from build123d import *

# Parameters (mm, degrees)
SKETCH1_W            = 94
SKETCH1_H            = 190
PLATE_DEPTH          = 12
SKETCH2_R            = 17.5
BOSS_DEPTH           = 10
SKETCH3_R            = 11
CENTER_HOLE_DEPTH    = 23
FILLET_R5_R          = 5
FILLET_R2_R          = 2
LPATTERN1_COUNT      = 5
LPATTERN1_PITCH      = 40
LPATTERN1_COUNT_DIR2 = 2
LPATTERN1_PITCH_DIR2 = 70
LPATTERN2_COUNT      = 2
LPATTERN2_PITCH      = 35


with BuildPart() as part:
    # Sketch1 → plate (new body)
    with BuildSketch(Plane(origin=(0, 0, 0), x_dir=(1, 0, 0), z_dir=(0, 1, 0))):
        Rectangle(SKETCH1_W, SKETCH1_H)
    extrude(amount=PLATE_DEPTH)

    # Sketch2 → boss (add)
    with BuildSketch(Plane(origin=(0, 12, 0), x_dir=(-1, 0, 0), z_dir=(0, 1, 0))):
        Circle(SKETCH2_R)
    extrude(amount=BOSS_DEPTH)

    # Sketch3 → center hole (cut, through all)
    with BuildSketch(Plane(origin=(0, 22, 0), x_dir=(-1, 0, 0), z_dir=(0, 1, 0))):
        Circle(SKETCH3_R)
    extrude(amount=-CENTER_HOLE_DEPTH, mode=Mode.SUBTRACT)

    # Sketch4 → pattern hole (revolve, cut)
    with BuildSketch(Plane(origin=(-35, 12, 80), x_dir=(0, 0, 1), z_dir=(1, 0, 0))):
        Polygon((0, 0), (0, 12), (4, 12), (4, 6.201721238), (6, 5), (6, 0), align=None)
    pattern_hole = revolve(axis=Axis((-35, 18.130023899, 80), (0, -1, 0)), mode=Mode.SUBTRACT)

    # Fillet R5
    fillet_r5_edges = [part.edges().sort_by_distance(p)[0] for p in [
        (-47, 6, -95),
        (47, 6, -95),
        (47, 6, 95),
        (-47, 6, 95),
    ]]
    fillet(fillet_r5_edges, radius=FILLET_R5_R)

    # Fillet R2
    fillet_r2_edges = [part.edges().sort_by_distance(p)[0] for p in [
        (17.5, 12, 0),
        (17.5, 22, 0),
        (47, 12, 0),
        (0, 12, 95),
        (-47, 12, 0),
        (0, 12, -95),
        (45.535533906, 12, -93.535533906),
        (-45.535533906, 12, -93.535533906),
        (-45.535533906, 12, 93.535533906),
        (45.535533906, 12, 93.535533906),
    ]]
    fillet(fillet_r2_edges, radius=FILLET_R2_R)

    # LPattern1: pattern hole 5 × 2
    with Locations(*[(j * LPATTERN1_PITCH_DIR2, 0, -i * LPATTERN1_PITCH) for i in range(LPATTERN1_COUNT) for j in range(LPATTERN1_COUNT_DIR2) if (i, j) != (0, 0)]):
        add(pattern_hole, mode=Mode.SUBTRACT)

    # LPattern2: pattern hole ×2
    with Locations(*[(i * LPATTERN2_PITCH, 0, 0) for i in range(1, LPATTERN2_COUNT)]):
        add(pattern_hole, mode=Mode.SUBTRACT)

    # LPattern3 copy 1 sketch → LPattern3 copy 1 (revolve, cut)
    with BuildSketch(Plane(origin=(0, 12, -80), x_dir=(0, 0, 1), z_dir=(1, 0, 0))):
        Polygon((0, 0), (0, 12), (4, 12), (4, 6.201721238), (6, 5), (6, 0), align=None)
    revolve(axis=Axis((0, 18.130023899, -80), (0, -1, 0)), mode=Mode.SUBTRACT)

    # LPattern3 copy 2 sketch → LPattern3 copy 2 (revolve, cut)
    with BuildSketch(Plane(origin=(-35, 12, -80), x_dir=(0, 0, 1), z_dir=(1, 0, 0))):
        Polygon((0, 0), (0, 12), (4, 12), (4, 6.201721238), (6, 5), (6, 0), align=None)
    revolve(axis=Axis((-35, 18.130023899, -80), (0, -1, 0)), mode=Mode.SUBTRACT)


solid = part.part
Read the model definition and answer for the solid it produces. Units are mm, in the model's axes. A direction names the side the tool comes from. Give positions to 0.01 mm unless a question says otherwise; leave off trailing zeros. Loops run counter-clockwise (first coordinate to the right, second up) from the corner with the lowest first, then second, coordinate; pieces in that order, holes last. Notation, with made-up numbers: (3.5, 75) - (18.5, 75) arc R18 cw to (18.5, 100) - close; hole circle Ø3 at (47.5, 54.5). An arc over 180 degrees is marked (long way). Answer as CSV lines item,"result". Start each with the question number.
1) Find section C-C (z = -40). Write down the section's boundary in (x, y).
2) Which of the six approach directions +Z, -Z, +X, -X, +Y, -Y give full straight-line access (tool end or side, diameter ignored) to faces 4 (the face through (40.857, 9.535, -41.301)), 5 (the face through (31.034, 2.94, 39.479))?
3) Determine the mould class of faces 1 (the face through (-1, 12, -22)), 2 (the face through (31.034, 2.94, -40.521)), 3 (the face through (45, 5, 94)) for opening direction Z: released by +Z, released by -Z, zero draft, split by the parting line, or undercut.
4) Find section A-A (z = 0). State how many separate pieces and enclosed holes the cut face has, then the cut area to 3 significant figures.
5) Each of these flat-tipped pins is pushed along its axis until it touches: pin 1 Ø1.5 at (x, z) = (7, 54.5) entering from +Y; pin 2 Ø1 at (x, y) = (-25.5, 11.5) entering from +Z; pin 3 Ø2 at (x, y) = (10, 19.5) entering from -Z. Where does it stop, or does it pass through?
6) Straight lines are drawn through the part: L1, parallel to Z at x = 35, y = 9.65; L2, parallel to X at y = 4.55, z = -80; L3, parallel to Z at x = 0, y = 8. For each, find the intervals that lie inside material, in ascending order. Write a range as from..to.
Findings below:
1,outline,"(-47, 0) - (-39, 0) - (-39, 5.8) - (-41, 7) - (-41, 12) - (-45, 12) arc R2 ccw to (-47, 10) - close; (-31, 0) - (31, 0) - (31, 5.8) - (29, 7) - (29, 12) - (-29, 12) - (-29, 7) - (-31, 5.8) - close; (39, 0) - (47, 0) - (47, 10) arc R2 ccw to (45, 12) - (41, 12) - (41, 7) - (39, 5.8) - close"
2,face 4,"+Y"
2,face 5,"+Y, -Y"
3,face 1,"zero draft"
3,face 2,"undercut"
3,face 3,"released by +Z"
4,separate pieces,"4"
4,enclosed holes,"0"
4,area,"755 mm^2"
5,pin 1,"y = 12"
5,pin 2,"z = 94.73"
5,pin 3,"z = -15.01"
6,L1,"-95..-86, -74..-46, -34..-6, 6..34, 46..74, 86..95"
6,L2,"-47..-39, -31..-4, 4..31, 39..47"
6,L3,"-95..-86, -74..-11, 11..74, 86..95"
